```python
from build123d import *

# Parameters (mm, degrees)
SKETCH_1_R          = 62.5
SKETCH_1_R_2        = 39.5
SKETCH_1_R_3        = 2
SKETCH_1_R_4        = 1.4
EXTRUDE_1_DEPTH     = 30.5
SKETCH_2_R          = 54.5
CUT_EXTRUDE_1_DEPTH = 18
SKETCH_3_R          = 7
CUT_EXTRUDE_2_DEPTH = 18
SKETCH_4_R          = 42.625
CUT_EXTRUDE_3_DEPTH = 10


with BuildPart() as part:
    # 草图1 → 凸台-拉伸1 (new body)
    with BuildSketch(Plane.XY):
        with Locations(Location((0, 0, 0), (0, 0, 180))):
            Circle(SKETCH_1_R)
        with Locations(Location((0, 0, 0), (0, 0, 180))):
            Circle(SKETCH_1_R_2, mode=Mode.SUBTRACT)
        with Locations(Location((0, -52.5, 0), (0, 0, 180))):
            Circle(SKETCH_1_R_3, mode=Mode.SUBTRACT)
        with Locations(Location((-28.383642916, -44.165810474, 0), (0, 0, 180))):
            Circle(SKETCH_1_R_3, mode=Mode.SUBTRACT)
        with Locations(Location((-47.755679756, -21.809288183, 0), (0, 0, 180))):
            Circle(SKETCH_1_R_3, mode=Mode.SUBTRACT)
        with Locations(Location((-51.965625699, 7.471529009, 0), (0, 0, 180))):
            Circle(SKETCH_1_R_3, mode=Mode.SUBTRACT)
        with Locations(Location((-39.676852654, 34.380188532, 0), (0, 0, 180))):
            Circle(SKETCH_1_R_3, mode=Mode.SUBTRACT)
        with Locations(Location((-14.790959234, 50.373381115, 0), (0, 0, 180))):
            Circle(SKETCH_1_R_3, mode=Mode.SUBTRACT)
        with Locations(Location((14.790959234, 50.373381115, 0), (0, 0, 180))):
            Circle(SKETCH_1_R_3, mode=Mode.SUBTRACT)
        with Locations(Location((39.676852654, 34.380188532, 0), (0, 0, 180))):
            Circle(SKETCH_1_R_3, mode=Mode.SUBTRACT)
        with Locations(Location((51.965625699, 7.471529009, 0), (0, 0, 180))):
            Circle(SKETCH_1_R_3, mode=Mode.SUBTRACT)
        with Locations(Location((47.755679756, -21.809288183, 0), (0, 0, 180))):
            Circle(SKETCH_1_R_3, mode=Mode.SUBTRACT)
        with Locations(Location((28.383642916, -44.165810474, 0), (0, 0, 180))):
            Circle(SKETCH_1_R_3, mode=Mode.SUBTRACT)
        with Locations(Location((-31.625977228, 49.210981142, 0), (0, 0, 180))):
            Circle(SKETCH_1_R_4, mode=Mode.SUBTRACT)
        with Locations(Location((0, 58.497205922, 0), (0, 0, 180))):
            Circle(SKETCH_1_R_4, mode=Mode.SUBTRACT)
        with Locations(Location((31.625977228, 49.210981142, 0), (0, 0, 180))):
            Circle(SKETCH_1_R_4, mode=Mode.SUBTRACT)
        with Locations(Location((53.210930145, 24.300617558, 0), (0, 0, 180))):
            Circle(SKETCH_1_R_4, mode=Mode.SUBTRACT)
        with Locations(Location((57.901788711, -8.3250204, 0), (0, 0, 180))):
            Circle(SKETCH_1_R_4, mode=Mode.SUBTRACT)
        with Locations(Location((44.209238476, -38.307523204, 0), (0, 0, 180))):
            Circle(SKETCH_1_R_4, mode=Mode.SUBTRACT)
        with Locations(Location((16.480567392, -56.127658058, 0), (0, 0, 180))):
            Circle(SKETCH_1_R_4, mode=Mode.SUBTRACT)
        with Locations(Location((-16.480567392, -56.127658058, 0), (0, 0, 180))):
            Circle(SKETCH_1_R_4, mode=Mode.SUBTRACT)
        with Locations(Location((-44.209238476, -38.307523204, 0), (0, 0, 180))):
            Circle(SKETCH_1_R_4, mode=Mode.SUBTRACT)
        with Locations(Location((-57.901788711, -8.3250204, 0), (0, 0, 180))):
            Circle(SKETCH_1_R_4, mode=Mode.SUBTRACT)
        with Locations(Location((-53.210930145, 24.300617558, 0), (0, 0, 180))):
            Circle(SKETCH_1_R_4, mode=Mode.SUBTRACT)
    extrude(amount=EXTRUDE_1_DEPTH)

    # 草图2 → 切除-拉伸1 (cut)
    with BuildSketch(Plane.XY.offset(30.5)):
        Circle(SKETCH_2_R)
    extrude(amount=-CUT_EXTRUDE_1_DEPTH, mode=Mode.SUBTRACT)

    # 草图3 → 切除-拉伸2 (cut)
    with BuildSketch(Plane.XY.offset(30.5)):
        with Locations((-39.676852654, 34.380188532)):
            Circle(SKETCH_3_R)
        with Locations((-14.790959234, 50.373381115)):
            Circle(SKETCH_3_R)
        with Locations((14.790959234, 50.373381115)):
            Circle(SKETCH_3_R)
        with Locations((39.676852654, 34.380188532)):
            Circle(SKETCH_3_R)
        with Locations((51.965625699, 7.471529009)):
            Circle(SKETCH_3_R)
        with Locations((47.755679756, -21.809288183)):
            Circle(SKETCH_3_R)
        with Locations((28.383642916, -44.165810474)):
            Circle(SKETCH_3_R)
        with Locations((0, -52.5)):
            Circle(SKETCH_3_R)
        with Locations((-28.383642916, -44.165810474)):
            Circle(SKETCH_3_R)
        with Locations((-47.755679756, -21.809288183)):
            Circle(SKETCH_3_R)
        with Locations((-51.965625699, 7.471529009)):
            Circle(SKETCH_3_R)
    extrude(amount=-CUT_EXTRUDE_2_DEPTH, mode=Mode.SUBTRACT)

    # 草图4 → 切除-拉伸3 (cut)
    with BuildSketch(Plane(origin=(0, 0, 0), x_dir=(-1, 0, 0), z_dir=(0, 0, -1))):
        Circle(SKETCH_4_R)
    extrude(amount=-CUT_EXTRUDE_3_DEPTH, mode=Mode.SUBTRACT)


solid = part.part
```
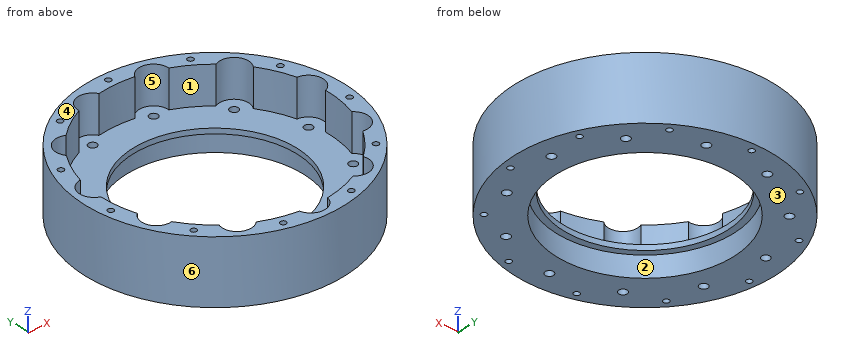
Design review of the part built by this model. Coordinates are the model's own, in mm. Face numbers are marked on the shaded views. A direction names the side the tool comes from. Coordinates: 2 decimals unless noted, no trailing zeros.
Q1. We need section A-A on z = 3.5. State how many separate pieces and enclosed holes the cut face has, and give its area (3 significant figures).
Reported:
separate pieces: 1
enclosed holes: 23
area: 6,360 mm2
Q2. Tool access review of the marked faces 1, 2 and 3: name each direction out of +Z, -Z, +X, -X, +Y, -Y from which nothing blocks a thin tool from reaching the whole face with its end or side.
Reported:
face 1: +Z
face 2: -Z
face 3: -Z, +X, -X, +Y, -Y
Q3. To check wall thickness, follow line 1 (Y direction, x = 0, z = 7.5) (3 decimals); line 2 (Y direction, x = -43.5, z = 21); line 3 (X direction, y = -55, z = 28.5). State the ranges of each line that lie inside material, in increasing order.
Reported:
line 1: y = -62.5 to -54.5, -50.5 to -42.625, 42.625 to 57.097, 59.897 to 62.5
line 2: y = -44.88 to -39.51, -37.1 to -32.83, 40.24 to 44.88
line 3: x = -29.69 to -17.31, -15.65 to -6.54, 6.54 to 15.65, 17.31 to 29.69
Q4. For pin 1 (4 mm diameter, centred on x = 4.5, z = 7.5, fed in from +Y); pin 2 (3 mm diameter, centred on x = -47, z = 10, fed in from -Y); pin 3 (1.5 mm diameter, centred on x = 45, z = 7.5, fed in from -Y), all flat-tipped, find the tip position at first contact; note any pin that passes through.
Reported:
pin 1: stops at y = 62.45
pin 2: stops at y = -42.85
pin 3: stops at y = -44.14
Q5. The part is to be moulded in two halves that separate along Y. For the marked faces 4, 5 and 6, say which applies: +Y half, -Y half, draft (parallel to the pull), parting line (faces both ways), or undercut.
Reported:
face 4: draft
face 5: undercut
face 6: parting line
